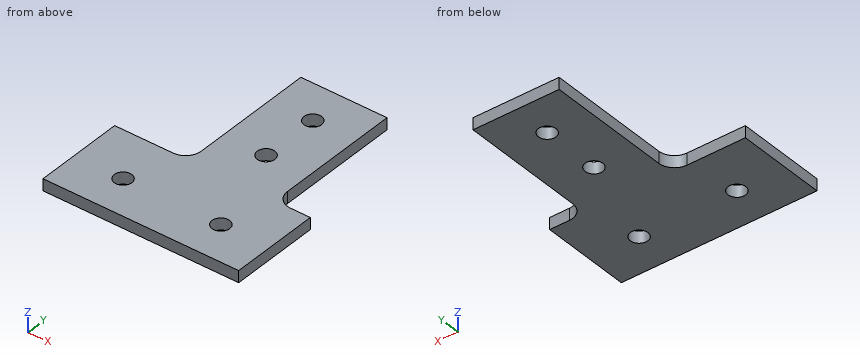
```python
from build123d import *

# Parameters (mm, degrees)
AUFSATZ_LINEAR_AUSTRAGEN1_DEPTH = 3
DURCHGANGSLOCH_F_R_M41_D        = 4.5
DURCHGANGSLOCH_F_R_M42_D        = 4.5
SKIZZE6_W                       = 22
SKIZZE6_H                       = 24
SCHNITT_LINEAR_AUSTRAGEN1_DEPTH = 76.80402364


with BuildPart() as part:
    # Skizze1 → Aufsatz-Linear austragen1 (new body)
    with BuildSketch(Plane.XY):
        with BuildLine():
            Line((-10.0526089, 11.5), (-25, 11.5))
            Line((-25, 11.5), (-25, -11.5))
            Line((-25, -11.5), (25, -11.5))
            Line((25, -11.5), (25, 11.5))
            Line((25, 11.5), (19.9473911, 11.5))
            ThreePointArc((19.9473911, 11.5), (17.118963975, 12.671572875), (15.9473911, 15.5))
            Line((15.9473911, 15.5), (15.9473911, 71.5))
            Line((15.9473911, 71.5), (-6.0526089, 71.5))
            Line((-6.0526089, 71.5), (-6.0526089, 15.5))
            ThreePointArc((-6.0526089, 15.5), (-7.224181775, 12.671572875), (-10.0526089, 11.5))
        make_face()
    extrude(amount=AUFSATZ_LINEAR_AUSTRAGEN1_DEPTH)

    # Durchgangsloch für M41 (through all)
    with Locations(Plane.XY.offset(3)):
        with Locations((4.9473911, 22.5), (4.9473911, 37.5)):
            Hole(DURCHGANGSLOCH_F_R_M41_D / 2)

    # Durchgangsloch für M42 (through all)
    with Locations(Plane.XY.offset(3)):
        with Locations((-12.5, -1.5), (12.5, -1.5)):
            Hole(DURCHGANGSLOCH_F_R_M42_D / 2)

    # Skizze6 → Schnitt-Linear austragen1 (cut, through all)
    with BuildSketch(Plane.XY.offset(3)):
        with Locations((4.9473911, 59.5)):
            Rectangle(SKIZZE6_W, SKIZZE6_H)
    extrude(amount=-SCHNITT_LINEAR_AUSTRAGEN1_DEPTH, mode=Mode.SUBTRACT)


solid = part.part
```
Design review of the part built by this model. Coordinates are the model's own, in mm. Give positions to 0.01 mm unless a question says otherwise; leave off trailing zeros. Loops run counter-clockwise (first coordinate to the right, second up) from the corner with the lowest first, then second, coordinate; pieces in that order, holes last. Notation, with made-up numbers: M -16,-11.75 L 26,-11.75 A27 ccw 26,4.25 Z; hole C 19.25,35.25 d6. An arc over 180 degrees is marked long. Return JSON: item names as keys, results as strings. Group by question number.
Item 1: We need section B-B (y = -1.5). Give the boundary of the cut face in (x, z), and give its area (3 significant figures).
Item 2: We need section A-A (x = 12.5). Give the boundary of the cut face in (y, z), and give its area (4 significant figures).
Item 3: We need section D-D (y = 22.5). Give the boundary of the cut face in (x, z).
Item 4: For probe 1 along Y at (x, z) = (12.5, 1.8); probe 2 along X at (y, z) = (-3, 1.95); probe 3 along Y at (x, z) = (-18.5, 0.75), list the stretches that pass through material, from the lowest coordinate up.
Item 5: We need section C-C (z = 0.6). Give the boundary of the cut face in (x, y), and give its area (3 significant figures).
Item 6: Insertion check: pin 1 Ø7 at (x, y) = (4.95, 37.5) entering from -Z; pin 2 Ø2.5 at (x, y) = (4.95, 22.5) entering from -Z; pin 3 Ø1 at (y, z) = (27.5, 1) entering from -X; pin 4 Ø0.9 at (x, z) = (-19, 1) entering from +Y. Each pin has a flat end and moves straight along its axis. Give the tip position at first contact, or say it passes through.
Output:
{
 "1": {"outline": "M -25,0 L -14.75,0 L -14.75,3 L -25,3 Z; M -10.25,0 L 10.25,0 L 10.25,3 L -10.25,3 Z; M 14.75,0 L 25,0 L 25,3 L 14.75,3 Z", "area": "123 mm^2"},
 "2": {"outline": "M -11.5,0 L -3.75,0 L -3.75,3 L -11.5,3 Z; M 0.75,0 L 47.5,0 L 47.5,3 L 0.75,3 Z", "area": "163.5 mm^2"},
 "3": {"outline": "M -6.05,0 L 2.7,0 L 2.7,3 L -6.05,3 Z; M 7.2,0 L 15.95,0 L 15.95,3 L 7.2,3 Z"},
 "4": {"probe 1": "y = -11.5 to -3.75, 0.75 to 47.5", "probe 2": "x = -25 to -14.18, -10.82 to 10.82, 14.18 to 25", "probe 3": "y = -11.5 to 11.5"},
 "5": {"outline": "M -25,-11.5 L 25,-11.5 L 25,11.5 L 19.95,11.5 A4 cw 15.95,15.5 L 15.95,47.5 L -6.05,47.5 L -6.05,15.5 A4 cw -10.05,11.5 L -25,11.5 Z; hole C -12.5,-1.5 d4.5; hole C 4.95,22.5 d4.5; hole C 4.95,37.5 d4.5; hole C 12.5,-1.5 d4.5", "area": "1,890 mm^2"},
 "6": {"pin 1": "stops at z = 0", "pin 2": "passes through", "pin 3": "stops at x = -6.05", "pin 4": "stops at y = 11.5"}
}
